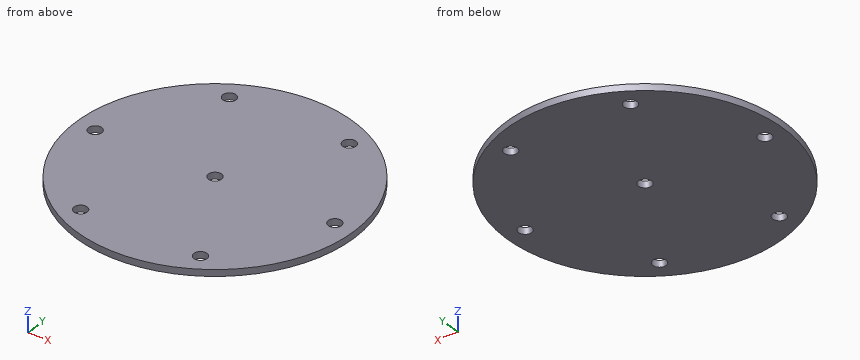
from build123d import *

# Parameters (mm, degrees)
F0_R     = 21
F1_DEPTH = 1
F2_D     = 2


# Not quite as in the source:
# - a feature names something its author has since deleted; it is built from what else it names


with BuildPart() as f1:
    # F0 (on Top) → F1 (new body)
    with BuildSketch(Plane.XY):
        Circle(F0_R)
    extrude(amount=F1_DEPTH)

    # F2 (through all)
    with Locations(Plane(origin=(0, 0, 0), x_dir=(1, 0, 0), z_dir=(0, 0, -1))):
        with Locations((-18, 0), (18, 0), (0, 0), (-9, 15.5884572681), (9, 15.5884572681), (9, -15.5884572681), (-9, -15.5884572681)):
            Hole(F2_D / 2)


solid = f1.part
Design review of the part built by this model. Coordinates are the model's own, in mm. Coordinates: 2 decimals unless noted, no trailing zeros. Order: outer loops, then holes, each group sorted by start corner. A loop starts at its lowest first (then second) coordinate and runs counter-clockwise, first axis right, second up. Notation, with made-up numbers: (71, 87) - (126, 87) arc R14 ccw to (126, 92) - close; hole circle Ø3 at (34, 15). An arc over 180 degrees is marked (long way). Put each result on its own line as item: value.
1) Take a section at B-B, the plane z = 0.5. Give the boundary of the cut face in (x, y), and give its area (3 significant figures).
Response values:
outline: circle Ø42 at (0, 0); hole circle Ø2 at (-18, 0); hole circle Ø2 at (-9, -15.59); hole circle Ø2 at (-9, 15.59); hole circle Ø2 at (0, 0); hole circle Ø2 at (9, -15.59); hole circle Ø2 at (9, 15.59); hole circle Ø2 at (18, 0)
area: 1,360 mm²
2) Take a section at D-D, the plane y = -11. Give the boundary of the cut face in (x, z), and give its area (3 significant figures).
Response values:
outline: (-17.89, 0) - (17.89, 0) - (17.89, 1) - (-17.89, 1) - close
area: 35.8 mm²
3) Wall thickness on L1, parallel to Y at x = 0, z = 0.4; L2, parallel to Y at x = 9, z = 0.5; L3, parallel to Y at x = 18, z = 0.15: over which ranges is each line inside the solid? List them lowest first. Write a range as from..to.
Response values:
L1: y = -21..-1, 1..21
L2: y = -18.97..-16.59, -14.59..14.59, 16.59..18.97
L3: y = -10.82..-1, 1..10.82
4) Take a section at C-C, the plane x = 18. Give the boundary of the cut face in (y, z), and give its area (3 significant figures).
Response values:
outline: (-10.82, 0) - (-1, 0) - (-1, 1) - (-10.82, 1) - close; (1, 0) - (10.82, 0) - (10.82, 1) - (1, 1) - close
area: 19.6 mm²
5) Take a section at A-A, the plane x = 9. Give the boundary of the cut face in (y, z), and give its area (3 significant figures).
Response values:
outline: (-18.97, 0) - (-16.59, 0) - (-16.59, 1) - (-18.97, 1) - close; (-14.59, 0) - (14.59, 0) - (14.59, 1) - (-14.59, 1) - close; (16.59, 0) - (18.97, 0) - (18.97, 1) - (16.59, 1) - close
area: 33.9 mm²
6) Insertion check: P1, Ø1.2, axis at x = 18, y = 0, coming from the +Z side. The pin has a flat end and moves straight along its axis. Give the tip position at first contact, or say it passes through.
Response values:
P1: passes through
